Read the model definition and answer for the solid it produces. Units are mm, in the model's axes. Round coordinates to 2 decimals unless told otherwise and drop trailing zeros. Loops run counter-clockwise (first coordinate to the right, second up) from the corner with the lowest first, then second, coordinate; pieces in that order, holes last. Notation, with made-up numbers: M -21,76 L 7,76 A10 ccw 7,82 Z; hole C -25.75,11 d5. An arc over 180 degrees is marked long. Write each question's results on one line, items separated by ' | '.
```python
from build123d import *

# Parameters (mm, degrees)
F0_R     = 56.5
F0_R_2   = 5
F0_R_3   = 35
F1_DEPTH = 4
F2_ANGLE = -15
F3_R     = 4.5
F4_DEPTH = 4


with BuildPart() as f1:
    # F0 (on Front) → F1 (new body)
    with BuildSketch(Plane.XZ):
        Circle(F0_R)
        with Locations((-38.971143, -22.5)):
            Circle(F0_R_2, mode=Mode.SUBTRACT)
        with Locations((38.971143, -22.5)):
            Circle(F0_R_2, mode=Mode.SUBTRACT)
        Circle(F0_R_3, mode=Mode.SUBTRACT)
        with Locations((0, 45)):
            Circle(F0_R_2, mode=Mode.SUBTRACT)
    extrude(amount=F1_DEPTH)


with BuildPart() as f1_1:
    # F2: moved
    add(f1.part.rotate(Axis((0, -4, 0), (0, -1, 0)), F2_ANGLE))

    # F3 (on face) → F4 (join)
    with BuildSketch(Plane.XZ.offset(4)):
        with BuildLine():
            Line((-56.5, 123), (-56.5, 0))
            ThreePointArc((-56.5, 0), (0, 56.5), (56.5, 0))
            Line((56.5, 0), (56.5, 73.5))
            ThreePointArc((56.5, 73.5), (53.068627, 83.710308), (44.167387, 89.776001))
            ThreePointArc((44.167387, 89.776001), (49.10698, 86.134844), (50.98986, 80.294265))
            ThreePointArc((50.98986, 80.294265), (34.214658, 72.939223), (40.17053, 90.260643))
            ThreePointArc((40.17053, 90.260643), (15.244627, 92.860772), (-8.158831, 101.824001))
            ThreePointArc((-8.158831, 101.824001), (-20.738354, 108.890352), (-31.308753, 118.710962))
            ThreePointArc((-31.308753, 118.710962), (-31.069903, 117.468456), (-30.98986, 116.205735))
            ThreePointArc((-30.98986, 116.205735), (-47.743504, 108.830893), (-41.867518, 126.167146))
            ThreePointArc((-41.867518, 126.167146), (-49.310618, 125.169671), (-56.5, 123))
        make_face()
        with BuildLine():
            ThreePointArc((-40.98986, 126.205735), (-41.428779, 126.18849), (-41.867518, 126.167146))
            ThreePointArc((-41.867518, 126.167146), (-47.743504, 108.830893), (-30.98986, 116.205735))
            ThreePointArc((-30.98986, 116.205735), (-31.069903, 117.468456), (-31.308753, 118.710962))
            ThreePointArc((-31.308753, 118.710962), (-34.86827, 124.113082), (-40.98986, 126.205735))
        make_face()
        with Locations((-40.98986, 116.205735)):
            Circle(F3_R, mode=Mode.SUBTRACT)
        with BuildLine():
            ThreePointArc((50.98986, 80.294265), (49.10698, 86.134844), (44.167387, 89.776001))
            ThreePointArc((44.167387, 89.776001), (42.996926, 90.060352), (41.809189, 90.260643))
            ThreePointArc((41.809189, 90.260643), (40.98986, 90.294265), (40.17053, 90.260643))
            ThreePointArc((40.17053, 90.260643), (34.214658, 72.939223), (50.98986, 80.294265))
        make_face()
        with Locations((40.98986, 80.294265)):
            Circle(F3_R, mode=Mode.SUBTRACT)
    extrude(amount=-F4_DEPTH)


solid = f1_1.part
```
1. Find section A-A, the plane z = -4. Give the vertices of the cut face in (x, y).
Completed:
outline: M -56.36,-4 L -34.77,-4 L -34.77,0 L -56.36,0 Z; M 34.77,-4 L 56.36,-4 L 56.36,0 L 34.77,0 Z
2. Find the intervals of material crossed by L1, parallel to Z at x = 14.5, y = -0.9; L2, parallel to X at y = -0.2, z = -16; L3, parallel to X at y = -3.75, z = 43, in increasing order.
Completed:
L1: z = -54.61 to -31.86, 31.86 to 39.36, 47.57 to 93.04 | L2: x = -54.19 to -45.93, -41.01 to -31.13, 31.13 to 54.19 | L3: x = -56.5 to 6.67, 16.63 to 56.5
3. Determine the mould class of faces 1 (the face through (-20.57, -2.03, 108.77)), 2 (the face through (-3, -4, 50)), 3 (the face through (-32.34, -1.97, -13.38)) for opening direction X: released by +X, released by -X, zero draft, split by the parting line, or undercut.
Completed:
face 1: released by +X | face 2: zero draft | face 3: undercut
4. Find section B-B, the plane x = -29. Give the vertices of the cut face in (y, z).
Completed:
outline: M -4,-48.49 L 0,-48.49 L 0,-19.6 L -4,-19.6 Z; M -4,19.6 L 0,19.6 L 0,116.14 L -4,116.14 Z
5. Find section C-C, the plane y = -2.9. Give the vertices of the cut face in (x, z).
Completed:
outline: M -56.5,0 A56.5 ccw 56.5,0 L 56.5,73.5 A16.91 ccw 44.17,89.78 A16.91 ccw 41.81,90.26 A10 ccw 40.17,90.26 A95.99 cw -8.16,101.82 A61.06 cw -31.31,118.71 A10 ccw -40.99,126.21 A47.03 ccw -41.87,126.17 A47.02 ccw -56.5,123 Z; hole C -43.47,-11.65 d10; hole C -40.99,116.21 d9; hole C 0,0 d70; hole C 11.65,43.47 d10; hole C 31.82,-31.82 d10; hole C 40.99,80.29 d9
6. Given P1, Ø1.5, axis at x = -25, y = -1.5, coming from the -Z side, flat-ended and moving along its own axis, determine where the tip first touches the part or whether it passes through.
Completed:
P1: stops at z = -51.03
7. Find section D-D, the plane x = 48. Give the vertices of the cut face in (y, z).
Completed:
outline: M -4,-29.8 L 0,-29.8 L 0,88.17 L -4,88.17 Z
